from build123d import *

# Parameters (mm, degrees)
SKETCH1_R           = 7.5
SKETCH1_R_2         = 5.25
BOSS_EXTRUDE1_DEPTH = 50
SKETCH2_R           = 2.5
CUT_EXTRUDE1_DEPTH  = 50


with BuildPart() as part:
    # Sketch1 → Boss-Extrude1 (new body)
    with BuildSketch(Plane(origin=(0, 0, 0), x_dir=(1, 0, 0), z_dir=(0, 1, 0))):
        with BuildLine():
            Line((-20, 40.822928267), (40, 40.822928267))
            Line((40, 40.822928267), (40, -39.177071733))
            Line((40, -39.177071733), (-20, -39.177071733))
            ThreePointArc((-20, -39.177071733), (-35.165750888, -32.215476544), (-39.773719933, -16.177071733))
            Line((-39.773719933, -16.177071733), (-57.320508076, -16.177071733))
            Line((-57.320508076, -16.177071733), (-57.320508076, -9.177071733))
            Line((-57.320508076, -9.177071733), (-37.320508076, -9.177071733))
            ThreePointArc((-37.320508076, -9.177071733), (0, 0.822928267), (-37.320508076, 10.822928267))
            Line((-37.320508076, 10.822928267), (-57.320508076, 10.822928267))
            Line((-57.320508076, 10.822928267), (-57.320508076, 17.822928267))
            Line((-57.320508076, 17.822928267), (-39.773719933, 17.822928267))
            ThreePointArc((-39.773719933, 17.822928267), (-35.165750888, 33.861333077), (-20, 40.822928267))
        make_face()
        with Locations(Location((20, 25.822928267, 0), (0, 0, 270))):
            Circle(SKETCH1_R, mode=Mode.SUBTRACT)
        with Locations(Location((20, -24.177071733, 0), (0, 0, 90))):
            Circle(SKETCH1_R, mode=Mode.SUBTRACT)
        with Locations(Location((30, 0.822928267, 0), (0, 0, 270))):
            Circle(SKETCH1_R_2, mode=Mode.SUBTRACT)
    extrude(amount=BOSS_EXTRUDE1_DEPTH)

    # Sketch2 → Cut-Extrude1 (cut)
    with BuildSketch(Plane.XY.offset(16.177071733)):
        with Locations((-48.547114004, 40)):
            Circle(SKETCH2_R)
        with Locations((-48.547114004, 25)):
            Circle(SKETCH2_R)
        with Locations((-48.547114004, 10)):
            Circle(SKETCH2_R)
    extrude(amount=-CUT_EXTRUDE1_DEPTH, mode=Mode.SUBTRACT)


solid = part.part
Source: CAD feature listing. Evaluate the final solid. Frame: model axes, mm. A direction names the side the tool comes from. Give positions to 0.01 mm unless a question says otherwise; leave off trailing zeros. Order: outer loops, then holes, each group sorted by start corner. A loop starts at its lowest first (then second) coordinate and runs counter-clockwise, first axis right, second up. Notation, with made-up numbers: (-13, 73.5) -> (18, 73.5) arc R31 cw to (18, 102.5) -> close; hole circle Ø1 at (79, 84.5). An arc over 180 degrees is marked (long way). Write item = value, one per line.
Q1. Cut plane A-A, the plane y = 10. Output: boundary loops of the cut face in (x, z).
Data:
outline = (-57.32, -17.82) -> (-51.05, -17.82) -> (-51.05, -10.82) -> (-57.32, -10.82) -> close; (-57.32, 9.18) -> (-51.05, 9.18) -> (-51.05, 16.18) -> (-57.32, 16.18) -> close; (-46.05, -17.82) -> (-39.77, -17.82) arc R20 ccw to (-20, -40.82) -> (40, -40.82) -> (40, 39.18) -> (-20, 39.18) arc R20 ccw to (-39.77, 16.18) -> (-46.05, 16.18) -> (-46.05, 9.18) -> (-37.32, 9.18) arc R20 cw (long way) to (-37.32, -10.82) -> (-46.05, -10.82) -> close; hole circle Ø15 at (20, -25.82); hole circle Ø15 at (20, 24.18); hole circle Ø10.5 at (30, -0.82)
Q2. Set-up query: faces 1 (the face through (-45, 25, 9.177)), 2 (the face through (34.427, 24.65, 1.999)). Return all of +Z, -Z, +X, -X, +Y, -Y with unobstructed straight access to the full face (end or side cutting, diameter ignored); none if empty.
Data:
face_1 = -X, +Y, -Y
face_2 = +Y, -Y
Q3. Cut plane C-C, the plane y = 15. Output: boundary loops of the cut face in (x, z), and give its area (3 significant figures).
Data:
outline = (-57.32, -17.82) -> (-39.77, -17.82) arc R20 ccw to (-20, -40.82) -> (40, -40.82) -> (40, 39.18) -> (-20, 39.18) arc R20 ccw to (-39.77, 16.18) -> (-57.32, 16.18) -> (-57.32, 9.18) -> (-37.32, 9.18) arc R20 cw (long way) to (-37.32, -10.82) -> (-57.32, -10.82) -> close; hole circle Ø15 at (20, -25.82); hole circle Ø15 at (20, 24.18); hole circle Ø10.5 at (30, -0.82)
area = 4,760 mm^2
Q4. Pin query (flat end, axial travel): pin 1 (6 mm diameter, centred on x = -48.55, y = 10, fed in from -Z); pin 2 (13.5 mm diameter, centred on x = 30, z = -0.82, fed in from -Y); pin 3 (4.5 mm diameter, centred on x = -48.55, y = 25, fed in from +Z); pin 4 (8 mm diameter, centred on x = -48.55, y = 40, fed in from +Z). Return the tip coordinate at first contact, or that it passes through.
Data:
pin_1 = -17.82
pin_2 = 0
pin_3 = through
pin_4 = 16.18
Q5. Cut plane B-B, the plane z = -12. Output: boundary loops of the cut face in (x, y), and give its area (3 significant figures).
Data:
outline = (-57.32, 0) -> (-36.59, 0) -> (-36.59, 50) -> (-57.32, 50) -> close; (-3.41, 0) -> (40, 0) -> (40, 50) -> (-3.41, 50) -> close; hole circle Ø5 at (-48.55, 10); hole circle Ø5 at (-48.55, 25); hole circle Ø5 at (-48.55, 40)
area = 3,150 mm^2
Q6. Pull-direction query (Y, two-part tool) for faces 3 (the face through (3, 50, -1)), 4 (the face through (-46.24, 39.04, -14.27)), 5 (the face through (27.436, 24.65, -26.799)); classes: released by +Y, released by -Y, zero draft, split by the parting line, or undercut.
Data:
face_3 = released by +Y
face_4 = undercut
face_5 = zero draft
Q7. Cut plane D-D, the plane x = -18.5. Output: boundary loops of the cut face in (y, z), and give its area (3 significant figures).
Data:
outline = (0, -40.82) -> (50, -40.82) -> (50, -20.77) -> (0, -20.77) -> close; (0, 19.12) -> (50, 19.12) -> (50, 39.18) -> (0, 39.18) -> close
area = 2,010 mm^2
Q8. Material intervals for line 1 (Z direction, x = -51, y = 27); line 2 (Z direction, x = 31.5, y = 17.5); line 3 (X direction, y = 48.5, z = 31), sorted ascending. Write a range as from..to.
Data:
line_1 = -17.82..-10.82, 9.18..16.18
line_2 = -40.82..-5.85, 4.21..39.18
line_3 = -36.13..16.89, 23.11..40
